Source: CAD feature listing. Evaluate the final solid. Frame: model axes, mm. Face numbers are marked on the shaded views. Give positions to 0.01 mm unless a question says otherwise; leave off trailing zeros. Write each loop counter-clockwise with the first axis right and the second up, starting at its lowest first coordinate (ties: lowest second). Pieces come first, ordered by that corner, then holes. Notation, with made-up numbers: (-8.75, -12) -> (26.25, -12) arc R22 cw to (26.25, 20) -> close; hole circle Ø7 at (21, -11). An arc over 180 degrees is marked (long way). Write item = value, one per line.
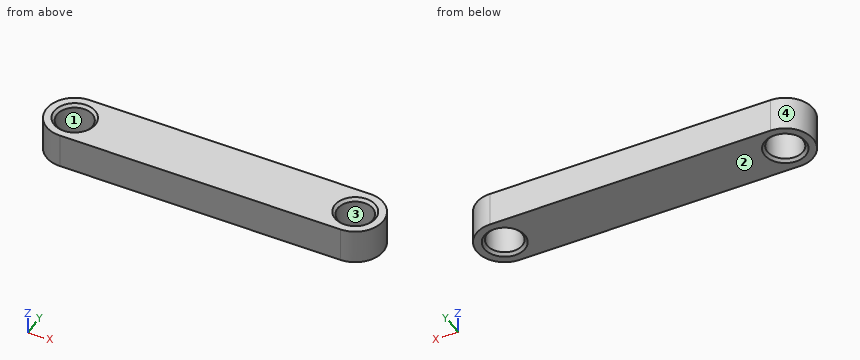
from build123d import *

# Parameters (mm, degrees)
BOSS_EXTRUDE1_DEPTH = 9.4615
SKETCH2_R           = 4.7625
SKETCH2_R_2         = 4.826
CUT_EXTRUDE1_DEPTH  = 10.4615
CHAMFER1_SIZE       = 0.762


with BuildPart() as part:
    # Sketch1 → Boss-Extrude1 (new body)
    with BuildSketch(Plane.XY):
        with BuildLine():
            Line((-38.1, 7.62), (38.1, 7.62))
            ThreePointArc((38.1, 7.62), (45.72, 0), (38.1, -7.62))
            Line((38.1, -7.62), (-38.1, -7.62))
            ThreePointArc((-38.1, -7.62), (-45.72, 0), (-38.1, 7.62))
        make_face()
    extrude(amount=BOSS_EXTRUDE1_DEPTH)

    # Sketch2 → Cut-Extrude1 (cut, through all)
    with BuildSketch(Plane.XY.offset(9.4615)):
        with Locations((38.1, 0)):
            Circle(SKETCH2_R)
        with Locations((-38.1, 0)):
            Circle(SKETCH2_R_2)
    extrude(amount=-CUT_EXTRUDE1_DEPTH, mode=Mode.SUBTRACT)

    # Chamfer1
    chamfer1_edges = [part.edges().sort_by_distance(p)[0] for p in [
        (33.3375, 0, 0),
        (33.3375, 0, 9.4615),
        (-42.926, 0, 0),
        (-42.926, 0, 9.4615),
    ]]
    chamfer(chamfer1_edges, length=CHAMFER1_SIZE)


solid = part.part
1) Cut plane A-A (y = 0). Return the cut outline in (x, z).
Computed:
outline = (-45.72, 0) -> (-43.69, 0) -> (-42.93, 0.76) -> (-42.93, 8.7) -> (-43.69, 9.46) -> (-45.72, 9.46) -> close; (-33.27, 0.76) -> (-32.51, 0) -> (32.58, 0) -> (33.34, 0.76) -> (33.34, 8.7) -> (32.58, 9.46) -> (-32.51, 9.46) -> (-33.27, 8.7) -> close; (42.86, 0.76) -> (43.62, 0) -> (45.72, 0) -> (45.72, 9.46) -> (43.62, 9.46) -> (42.86, 8.7) -> close
2) Draft query along Y for the marked faces 1, 2, 3 and 4. Return one class per face: pulls with the +Y half, pulls with the -Y half, needs draft (parallel to the pull), parting line crosses it, or undercut.
Computed:
face_1 = undercut
face_2 = needs draft
face_3 = undercut
face_4 = parting line crosses it
3) Material intervals for L1, parallel to X at y = -0.25, z = 4.25; L2, parallel to Y at x = -38.1, z = 4; L3, parallel to X at y = 2.25, z = 2.5, sorted ascending.
Computed:
L1 = -45.72 to -42.92, -33.28 to 33.34, 42.86 to 45.72
L2 = -7.62 to -4.83, 4.83 to 7.62
L3 = -45.38 to -42.37, -33.83 to 33.9, 42.3 to 45.38
4) Cut plane B-B (z = 6.75). Return the cut outline in (x, y) (1 decimal), then the cut area to 3 significant figures.
Computed:
outline = (-38.1, -7.6) -> (38.1, -7.6) arc R7.6 ccw to (38.1, 7.6) -> (-38.1, 7.6) arc R7.6 ccw to start; hole circle Ø9.7 at (-38.1, 0); hole circle Ø9.5 at (38.1, 0)
area = 1,200 mm²
